Build history of the part. All positions in model axes, mm. Face numbers are marked on the shaded views. Give positions to 0.01 mm unless a question says otherwise; leave off trailing zeros. Order: outer loops, then holes, each group sorted by start corner. A loop starts at its lowest first (then second) coordinate and runs counter-clockwise, first axis right, second up. Notation, with made-up numbers: (42.5, 63.25) - (77.5, 63.25) arc R31 cw to (77.5, 94.25) - close; hole circle Ø7 at (-27.5, 42.5). An arc over 180 degrees is marked (long way). Answer in a Markdown table with one row per item.
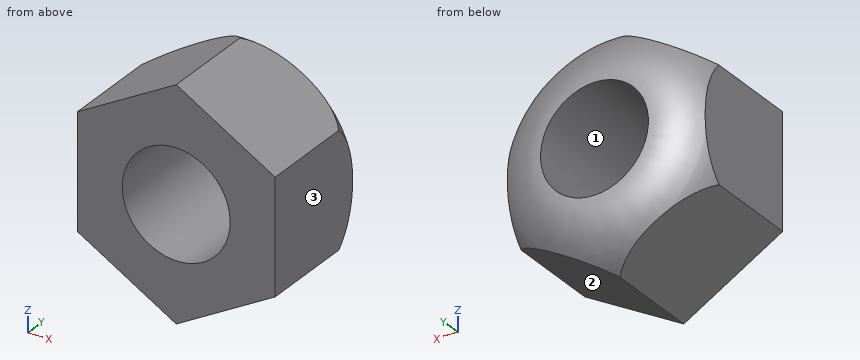
```python
from build123d import *

# Parameters (mm, degrees)
SKETCH3_R           = 1.5
BOSS_EXTRUDE1_DEPTH = 1.85


with BuildPart() as part:
    # Sketch3 → Boss-Extrude1 (new, symmetric)
    with BuildSketch(Plane(origin=(0, 0, 0), x_dir=(1, 0, 0), z_dir=(0, 1, 0))):
        Polygon((2.75, 1.58771324), (0, 3.175426481), (-2.75, 1.58771324), (-2.75, -1.58771324), (0, -3.175426481), (2.75, -1.58771324), align=None)
        with Locations(Location((0, 0, 0), (0, 0, 270))):
            Circle(SKETCH3_R, mode=Mode.SUBTRACT)
    extrude(amount=BOSS_EXTRUDE1_DEPTH, both=True)

    # Sketch5 → Cut-Revolve1 (revolve, cut)
    with BuildSketch(Plane(origin=(0, 0, 0), x_dir=(0, 0, -1), z_dir=(1, 0, 0))):
        with BuildLine():
            Line((1.5, 1.85), (3.175426481, 1.85))
            Line((3.175426481, 1.85), (3.175426481, 0.784503734))
            ThreePointArc((3.175426481, 0.784503734), (2.492765857, 1.561062444), (1.5, 1.85))
        make_face()
    revolve(axis=Axis((0, 0, 0), (0, 1, 0)), mode=Mode.SUBTRACT)


solid = part.part
```
1. Drop a flat-ended pin along its axis: P1, Ø2, axis at x = 1.5, y = -1, coming from the -Z side. Give the stop position or say it passes through.
Check result:
| item | result |
|---|---|
| P1 | stops at z = -2.89 |
2. Probe line 1 (X direction, y = 0.6, z = 0); line 2 (Z direction, x = 0.3, y = 0.2); line 3 (Z direction, x = -1.15, y = 0.55). List the from-to ranges inside material, lowest first.
Check result:
| item | result |
|---|---|
| line 1 | x = -2.75 to -1.5, 1.5 to 2.75 |
| line 2 | z = -3 to -1.47, 1.47 to 3 |
| line 3 | z = -2.51 to -0.96, 0.96 to 2.51 |
3. Cut at A-A on y = -1.45. Write the cut outline in (x, z).
Check result:
| item | result |
|---|---|
| outline | (-2.75, -1.59) - (0, -3.18) - (2.75, -1.59) - (2.75, 1.59) - (0, 3.18) - (-2.75, 1.59) - close; hole circle Ø3 at (0, 0) |
4. Two-plate mould, pull along Z, no slides. Class the marked faces 1, 2 and 3: +Z half, -Z half, draft (parallel to the pull), parting line (faces both ways), or undercut.
Check result:
| item | result |
|---|---|
| face 1 | undercut |
| face 2 | -Z half |
| face 3 | draft |
